Autodesk Inventor part; units mm, degrees
ref_plane "XZ Plane" through (0, 0, 0) normal (0, 1, 0) x (-1, 0, 0)
ref_plane "XY Plane" through (0, 0, 0) normal (0, 0, 1) x (1, 0, 0)
sketch "Sketch1" plane through (0, 0, 0) normal (0, 0, 1) x (1, 0, 0)
  line L0 (-38.1, -76.2) -> (38.1, -76.2)
  line L1 (38.1, -76.2) -> (38.1, 76.2)
  line L2 (38.1, 76.2) -> (-38.1, 76.2)
  line L3 (-38.1, 76.2) -> (-38.1, -76.2)
  line L4 (-38.1, -76.2) -> (38.1, 76.2) construction
  line L5 (38.1, -76.2) -> (-38.1, 76.2) construction
  point P0 (0, 0)
  dimension "d0" = 76.2
  dimension "d1" = 152.4
extrude "Extrusion1" add sketch "Sketch1" along normal mid plane 52.324
sketch "Sketch2" plane through (0, 0, 26.162) normal (0, 0, 1) x (1, 0, 0)
  line L0 (-38.1, -76.2) -> (38.1, -76.2)
  line L1 (38.1, -76.2) -> (38.1, 76.2)
  line L2 (38.1, 76.2) -> (-38.1, 76.2)
  line L3 (-38.1, 76.2) -> (-38.1, -76.2)
  circle A0 centre (0, 38.608) radius 23.495
  line L4 (-46.8851, 0) -> (67.5058, 0) construction
  circle A1 centre (0, -38.608) radius 23.495
  point P0 (0, 0)
  dimension "d4" = 46.99
  dimension "d8" = 38.608
extrude "Extrusion3" add sketch "Sketch2" along normal blind 4.826 contours A0 | A1
sketch "Sketch4" plane through (0, -38.608, 30.988) normal (0, 0, 1) x (1, 0, 0)
  circle A0 centre (0, 0) radius 23.495
  circle A1 centre (0, 0) radius 9.525
  point P0 (0, 38.608)
  dimension "d11" = 19.05
extrude "Extrusion4" add sketch "Sketch4" along normal blind 55.372 contours A1
sketch "Sketch5" plane through (0, 0, -26.162) normal (0, 0, -1) x (-1, 0, 0)
  circle A0 centre (0, 38.608) radius 23.495
  circle A1 centre (0, 38.608) radius 6.35
  point P0 (0, 0)
  dimension "d14" = 12.7
extrude "Extrusion5" cut sketch "Sketch5" against normal blind 52.324 contours A1
properties part number "A28-400-G Gearbox" material "Aluminum 6061"
Design review of the part built by this model. Coordinates are the model's own, in mm. A direction names the side the tool comes from. Round coordinates to 2 decimals unless told otherwise and drop trailing zeros. Loops run counter-clockwise (first coordinate to the right, second up) from the corner with the lowest first, then second, coordinate; pieces in that order, holes last. Notation, with made-up numbers: (-26, 28) - (15, 28) arc R19 ccw to (15, 47) - close; hole circle Ø8 at (-5, 71.25). An arc over 180 degrees is marked (long way). One line per item, written item: value. Start each with the question number.
1) Consider section A-A on x = 0. Give the boundary of the cut face in (y, z).
2) Consider section D-D on x = -18.5. Give the boundary of the cut face in (y, z), then the cut area to 3 significant figures.
3) Consider section C-C on x = 15. Give the boundary of the cut face in (y, z).
4) Insertion check: pin 1 Ø14 at (x, y) = (-1, 41) entering from -Z; pin 2 Ø8 at (x, y) = (0, 6) entering from +Z; pin 3 Ø2 at (x, z) = (7, 46.5) entering from -Y; pin 4 Ø3 at (y, z) = (-17.5, 31.5) entering from -X. Each pin has a flat end and moves straight along its axis. Give the tip position at first contact, or say it passes through.
5) Draft analysis for pull direction Y (two halves, no side actions). For faces 4 (the cylindrical face through (-1.24, -48.05, 58.29)), 5 (the flat face through (-1, 1, 26.162)), 6 (the flat face through (-1, 1, -26.162)), state which applies: +Y half, -Y half, draft (parallel to the pull), parting line (faces both ways), or undercut.
6) Consider section B-B on z = 28.5. Give the boundary of the cut face in (x, y) (3 decimals).
7) To check wall thickness, follow L1, parallel to Y at x = 0, z = 8; L2, parallel to Z at x = 6.5, y = 57; L3, parallel to Z at x = -22, y = -21.5. State the ranges of each line that lie inside material, in increasing order. Write a range as from..to.
8) For faces 1 (the flat face through (0, 39, 26.162)), 2 (the cylindrical face through (-3.059, -61.903, 28.541)), 3 (the flat face through (0, 39, 30.988)), list the 3-axis set-ups (+Z, -Z, +X, -X, +Y, -Y) from which the entire face can be reached by the end or side of a thin tool; tool diameter is ignored.
Reported:
1. outline: (-76.2, -26.16) - (32.26, -26.16) - (32.26, 26.16) - (44.96, 26.16) - (44.96, -26.16) - (76.2, -26.16) - (76.2, 26.16) - (62.1, 26.16) - (62.1, 30.99) - (15.11, 30.99) - (15.11, 26.16) - (-15.11, 26.16) - (-15.11, 30.99) - (-29.08, 30.99) - (-29.08, 86.36) - (-48.13, 86.36) - (-48.13, 30.99) - (-62.1, 30.99) - (-62.1, 26.16) - (-76.2, 26.16) - close
2. outline: (-76.2, -26.16) - (76.2, -26.16) - (76.2, 26.16) - (53.09, 26.16) - (53.09, 30.99) - (24.12, 30.99) - (24.12, 26.16) - (-24.12, 26.16) - (-24.12, 30.99) - (-53.09, 30.99) - (-53.09, 26.16) - (-76.2, 26.16) - close
2. area: 8,250 mm^2
3. outline: (-76.2, -26.16) - (76.2, -26.16) - (76.2, 26.16) - (56.69, 26.16) - (56.69, 30.99) - (20.52, 30.99) - (20.52, 26.16) - (-20.52, 26.16) - (-20.52, 30.99) - (-56.69, 30.99) - (-56.69, 26.16) - (-76.2, 26.16) - close
4. pin 1: stops at z = -26.16
4. pin 2: stops at z = 26.16
4. pin 3: stops at y = -46.01
4. pin 4: stops at x = -12.81
5. face 4: parting line
5. face 5: undercut
5. face 6: draft
6. outline: circle Ø46.99 at (0, -38.608); circle Ø46.99 at (0, 38.608)
7. L1: y = -76.2..32.26, 44.96..76.2
7. L2: z = -26.16..30.99
7. L3: z = -26.16..26.16
8. face 1: -Z
8. face 2: +Z
8. face 3: +Z, +X, -X, +Y
